Input: part model. Units: mm. Frame: model coordinates. A direction names the side the tool comes from. Give positions to 0.01 mm unless a question says otherwise; leave off trailing zeros. Write each loop counter-clockwise with the first axis right and the second up, starting at its lowest first coordinate (ties: lowest second). Pieces come first, ordered by that corner, then holes. Notation, with made-up numbers: (16.25, 7.5) -> (61.25, 7.5) arc R14 cw to (61.25, 31.5) -> close; hole circle Ø4 at (-21.5, 65.25). An arc over 180 degrees is marked (long way). Return JSON: item names as keys, results as strings. Group by question number.
Item 1: Line query: line 1 (Z direction, x = 24.9, y = -1.45); line 2 (Y direction, x = 3, z = 50.5); line 3 (Z direction, x = 24.9, y = -3.55). Output: solid intervals per line, ascending. Write a range as [from, to].
Item 2: Pin query (flat end, axial travel): P1, Ø10, axis at x = 21.5, y = 1.5, coming from the -Z side; P2, Ø11, axis at x = 26, z = 14.5, coming from the +Y side; P3, Ø11, axis at x = 44, y = 11, coming from the +Z side; P4, Ø8, axis at x = 24.9, z = 42.65, coming from the +Y side. Return the tip coordinate at first contact, or that it passes through.
Item 3: Set-up query: faces 1 (the face through (5, 20.7, 27)), 2 (the face through (50.8, 8, 28)), 3 (the face through (39.8, 21, 27)), 4 (the face through (25.98, -1.48, 7.77)), 5 (the face through (25, -5, 28)). Return all of +Z, -Z, +X, -X, +Y, -Y with unobstructed straight access to the full face (end or side cutting, diameter ignored); none if empty.
Item 4: Mould query, pull axis Z, two halves, no side actions, for faces 6 (the face through (23.053, -3.986, 11.884)), 7 (the face through (25, -3, 10)), 8 (the face through (-1, 9, 28)), 9 (the face through (20.9, -0.5, 55.3)). Classes: released by +Z, released by -Z, zero draft, split by the parting line, or undercut.
Item 5: Section D-D, the plane z = 33. Return loops of the section in (x, y).
Item 6: Section B-B, the plane y = 19.75. Return loops of the section in (x, z), then the cut area to 3 significant figures.
Item 7: Section C-C, the plane z = 42.65. Return loops of the section in (x, y), then the cut area to 3 significant figures.
Item 8: Section A-A, the plane x = 24.9. Return loops of the section in (y, z).
from build123d import *

# Parameters (mm, degrees)
PAD_DEPTH    = 55.3
PAD001_DEPTH = 1
SKETCH002_R  = 2
HOLE_DEPTH   = 25
SKETCH003_R  = 5
POCKET_DEPTH = 3


with BuildPart() as part:
    # Sketch → Pad (new body)
    with BuildSketch(Plane.XY):
        Polygon((0, 0), (0, 20.7), (10, 20.7), (10, 21.7), (-1, 21.7), (-1, -5), (50.8, -5), (50.8, 21.7), (39.8, 21.7), (39.8, 20.7), (49.8, 20.7), (49.8, 0), align=None)
    extrude(amount=PAD_DEPTH)

    # Sketch001 (on Face13 of Pad) → Pad001 (join)
    with BuildSketch(Plane(origin=(0, 0, 0), x_dir=(1, 0, 0), z_dir=(0, 0, -1))):
        Polygon((-1, 5), (50.8, 5), (50.8, -21.7), (39.8, -21.7), (39.8, 0), (10, 0), (10, -21.7), (-1, -21.7), align=None)
    extrude(amount=PAD001_DEPTH)

    # Sketch002 (on Face14 of Pad001) → Hole (cut)
    with BuildSketch(Plane(origin=(0, 0, 0), x_dir=(-1, 0, 0), z_dir=(0, 1, 0))):
        with Locations((-24.9, 42.65)):
            Circle(SKETCH002_R)
        with Locations((-24.9, 12.65)):
            Circle(SKETCH002_R)
    extrude(amount=-HOLE_DEPTH, mode=Mode.SUBTRACT)

    # Sketch003 (on Face14 of Pad001) → Pocket (cut)
    with BuildSketch(Plane(origin=(0, 0, 0), x_dir=(-1, 0, 0), z_dir=(0, 1, 0))):
        with Locations((-24.9, 42.65)):
            Circle(SKETCH003_R)
        with Locations((-24.9, 12.65)):
            Circle(SKETCH003_R)
    extrude(amount=-POCKET_DEPTH, mode=Mode.SUBTRACT)


solid = part.part
Answer below:
{
 "1": {"line 1": "z = [-1, 7.65], [17.65, 37.65], [47.65, 55.3]", "line 2": "y = [-5, 0], [20.7, 21.7]", "line 3": "z = [-1, 10.65], [14.65, 40.65], [44.65, 55.3]"},
 "2": {"P1": "stops at z = -1", "P2": "stops at y = 0", "P3": "stops at z = 0", "P4": "stops at y = -3"},
 "3": {"face 1": "+Z", "face 2": "+Z, -Z, +X, +Y, -Y", "face 3": "+Z, -Z, +Y", "face 4": "+Y", "face 5": "+Z, -Z, +X, -X, -Y"},
 "4": {"face 6": "undercut", "face 7": "undercut", "face 8": "zero draft", "face 9": "released by +Z"},
 "5": {"outline": "(-1, -5) -> (50.8, -5) -> (50.8, 21.7) -> (39.8, 21.7) -> (39.8, 20.7) -> (49.8, 20.7) -> (49.8, 0) -> (0, 0) -> (0, 20.7) -> (10, 20.7) -> (10, 21.7) -> (-1, 21.7) -> close"},
 "6": {"outline": "(-1, -1) -> (10, -1) -> (10, 0) -> (0, 0) -> (0, 55.3) -> (-1, 55.3) -> close; (39.8, -1) -> (50.8, -1) -> (50.8, 55.3) -> (49.8, 55.3) -> (49.8, 0) -> (39.8, 0) -> close", "area": "133 mm2"},
 "7": {"outline": "(-1, -5) -> (22.9, -5) -> (22.9, -3) -> (19.9, -3) -> (19.9, 0) -> (0, 0) -> (0, 20.7) -> (10, 20.7) -> (10, 21.7) -> (-1, 21.7) -> close; (26.9, -5) -> (50.8, -5) -> (50.8, 21.7) -> (39.8, 21.7) -> (39.8, 20.7) -> (49.8, 20.7) -> (49.8, 0) -> (29.9, 0) -> (29.9, -3) -> (26.9, -3) -> close", "area": "284 mm2"},
 "8": {"outline": "(-5, -1) -> (0, -1) -> (0, 7.65) -> (-3, 7.65) -> (-3, 10.65) -> (-5, 10.65) -> close; (-5, 14.65) -> (-3, 14.65) -> (-3, 17.65) -> (0, 17.65) -> (0, 37.65) -> (-3, 37.65) -> (-3, 40.65) -> (-5, 40.65) -> close; (-5, 44.65) -> (-3, 44.65) -> (-3, 47.65) -> (0, 47.65) -> (0, 55.3) -> (-5, 55.3) -> close"}
}
